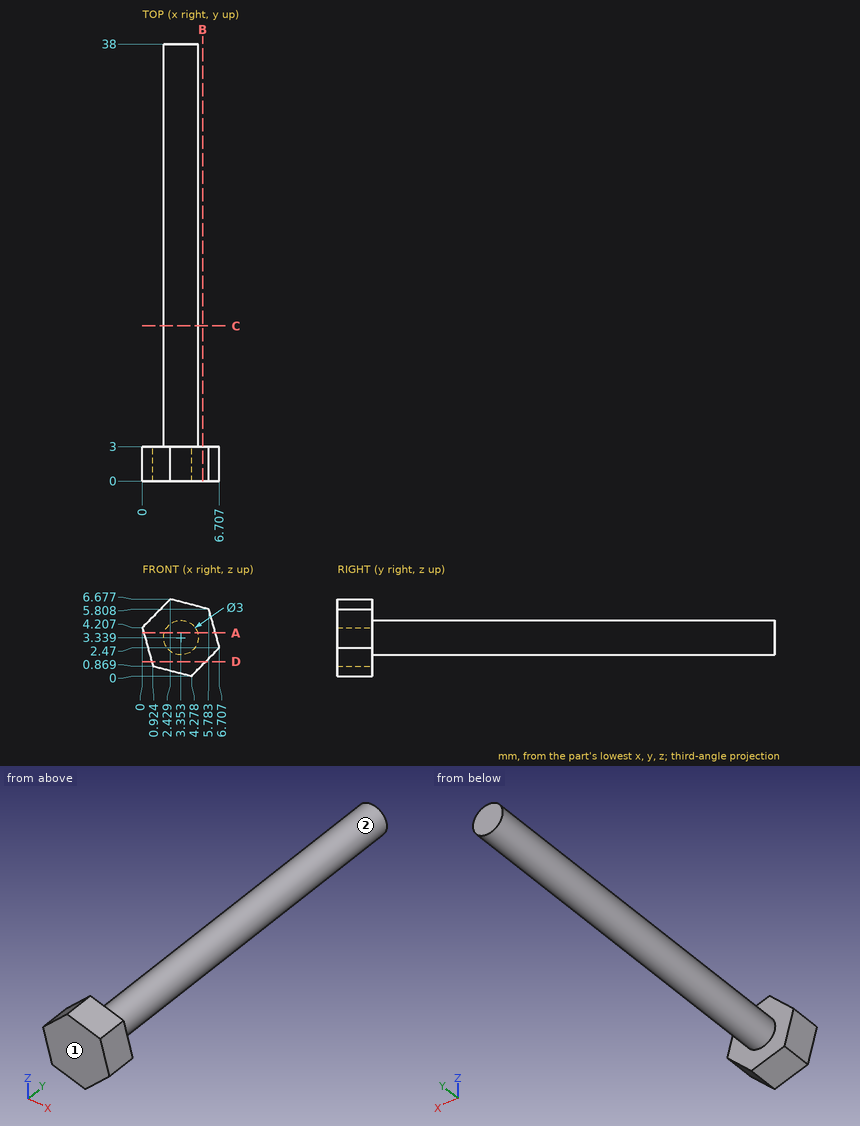
Study the drawing (mm; zero at the part's minimum x, y, z) and answer. A direction names the side the tool comes from. Give positions to 0.01 mm unless a question says otherwise; leave off trailing zeros. Write each loop counter-clockwise with the first axis right and the second up, starting at its lowest first coordinate (ties: lowest second). Pieces come first, ordered by that corner, then holes. Notation, with made-up numbers: (55.5, -34.5) -> (96.5, -34.5) arc R8 cw to (96.5, -23.5) -> close; hole circle Ø6 at (62, 45.25). An arc over 180 degrees is marked (long way). Write item = value, one per line.
Q1. Section D-D on z = 1.25 is taken. Determine the outline of the cut face in (x, y), and give its area (3 significant figures).
Computed values:
outline = (0.82, 0) -> (5.51, 0) -> (5.51, 3) -> (0.82, 3) -> close
area = 14.1 mm^2
Q2. Consider line 1 along Y through (x, z) = (5, 2.5); line 2 along Z through (x, y) = (3.5, 3.5) (1 decimal); line 3 along Z through (x, y) = (4, 9.5) (1 decimal). Determine where each line is inside the solid, lowest interval first.
Computed values:
line_1 = 0 to 3
line_2 = 1.8 to 4.8
line_3 = 2 to 4.7
Q3. Section A-A on z = 3.75 is taken. Determine the outline of the cut face in (x, y) (1 decimal).
Computed values:
outline = (0.1, 0) -> (6.4, 0) -> (6.4, 3) -> (4.8, 3) -> (4.8, 38) -> (1.9, 38) -> (1.9, 3) -> (0.1, 3) -> close
Q4. A tool of negligible diameter and unlimited length cuts with its end or side. For the marked faces 1 and 2, from which of +Z, -Z, +X, -X, +Y, -Y can it reach the whole face along a straight path? Write none if from no direction.
Computed values:
face_1 = +Z, -Z, +X, -X, -Y
face_2 = +Y
Q5. Section C-C on y = 13.5 is taken. Determine the outline of the cut face in (x, z).
Computed values:
outline = circle Ø3 at (3.35, 3.34)
Q6. Flat-ended cylindrical pins translate along their axes: pin 1 Ø4 at (y, z) = (19, 2) entering from +X; pin 2 Ø4 at (y, z) = (31, 5.5) entering from -X. Find the tip coordinate at first contact, or state that the pin passes through.
Computed values:
pin_1 = 4.85
pin_2 = 1.86
Q7. Section B-B on x = 5.25 is taken. Determine the outline of the cut face in (y, z).
Computed values:
outline = (0, 0.99) -> (3, 0.99) -> (3, 5.95) -> (0, 5.95) -> close
